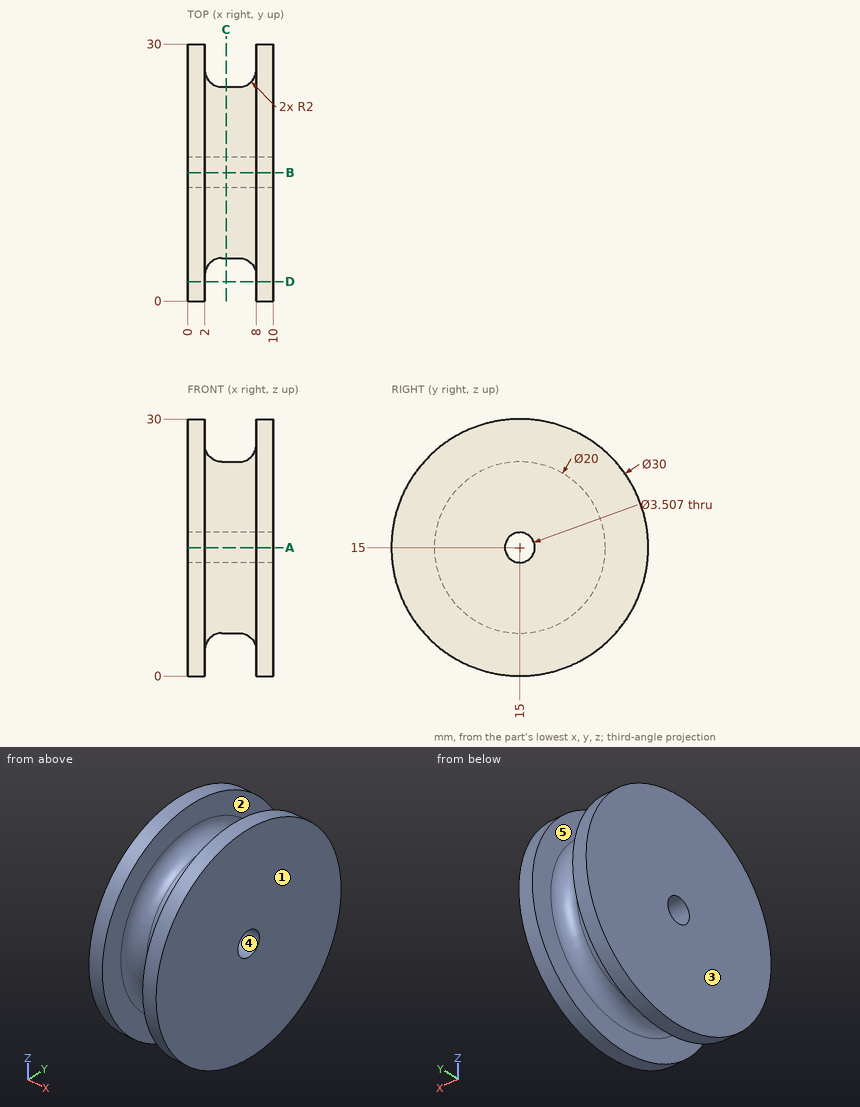
Geometry: see drawing. Coordinates: mm, zero at the bounding-box minimum. A direction names the side the tool comes from. Round coordinates to 2 decimals unless told otherwise and drop trailing zeros. Loops run counter-clockwise (first coordinate to the right, second up) from the corner with the lowest first, then second, coordinate; pieces in that order, holes last. Notation, with made-up numbers: M 86.25,53 L 128.25,53 A14 ccw 128.25,76 Z; hole C 32,55.5 d3. An arc over 180 degrees is marked long. Use a Markdown table: item, result. Add a question column.
1. Set-up query: the marked faces 4 and 5. Return all of +Z, -Z, +X, -X, +Y, -Y with unobstructed straight access to the full face (end or side cutting, diameter ignored); none if empty.
2. Pull-direction query (X, two-part tool) for the marked faces 1, 2 and 3; classes: +X half, -X half, draft (parallel to the pull), parting line (faces both ways), or undercut.
3. Ray query, line 1 along X through (y, z) = (19, 26.25); line 2 along Z through (x, y) = (4, 15); line 3 along Z through (x, y) = (6.5, 15). Return the intervals inside material, ascending. Write a range as [from, to].
4. Cut plane D-D, the plane y = 2.25. Output: boundary loops of the cut face in (x, z), and give its area (3 significant figures).
5. Cut plane A-A, the plane z = 15. Output: boundary loops of the cut face in (x, y).
6. Cut plane C-C, the plane x = 4.5. Output: boundary loops of the cut face in (y, z).
7. Contact query for flat-ended pins moving along their axis: pin 1 (1 mm diameter, centred on x = 8, z = 26, fed in from -Y); pin 2 (5 mm diameter, centred on x = 2, z = 20, fed in from -Y); pin 3 (1.5 mm diameter, centred on x = 7.5, y = 13.5, fed in from -Z); pin 4 (3 mm diameter, centred on y = 15, z = 15, fed in from -X). Output: stop coordinate, or through.
Solution:
| question | item | result |
|---|---|---|
| 1 | face 4 | +X, -X |
| 1 | face 5 | none |
| 2 | face 1 | +X half |
| 2 | face 2 | undercut |
| 2 | face 3 | -X half |
| 3 | line 1 | x = [0, 2], [8, 10] |
| 3 | line 2 | z = [5, 13.25], [16.75, 25] |
| 3 | line 3 | z = [4.94, 13.25], [16.75, 25.06] |
| 4 | outline | M 0,7.1 L 2,7.1 L 2,22.9 L 0,22.9 Z; M 8,7.1 L 10,7.1 L 10,22.9 L 8,22.9 Z |
| 4 | area | 63.2 mm2 |
| 5 | outline | M 0,0 L 2,0 L 2,3 A2 cw 4,5 L 6,5 A2 cw 8,3 L 8,0 L 10,0 L 10,13.25 L 0,13.25 Z; M 0,16.75 L 10,16.75 L 10,30 L 8,30 L 8,27 A2 cw 6,25 L 4,25 A2 cw 2,27 L 2,30 L 0,30 Z |
| 6 | outline | C 15,15 d20; hole C 15,15 d3.51 |
| 7 | pin 1 | stops at y = 4.29 |
| 7 | pin 2 | stops at y = 0.21 |
| 7 | pin 3 | stops at z = 0.03 |
| 7 | pin 4 | passes through |
